Solid Edge part; units mm, degrees
sketch "Sketch1" plane through (0, 0, 0) normal (0, 0, 1) x (1, 0, 0)
  line L0 (40, -40) -> (40, 40)
  line L1 (40, 40) -> (-40, 40)
  line L2 (-40, 40) -> (-40, -40)
  line L3 (-40, -40) -> (40, -40)
extrude "Protrusion1" add sketch "Sketch1" along normal blind 700
extrude "Extrusionsausschnitt_1" [suppressed]
sketch "Sketch2" plane through (40, 0, 350) normal (1, 0, 0) x (0, 0, 1)
  circle A0 centre (250, 79.99) radius 60
  circle A1 centre (250, 79.99) radius 41.1
extrude "Protrusion2" add sketch "Sketch2" against normal up to vertex (80 mm away)
sketch "Sketch3" plane through (40, -55, 350) normal (1, 0, 0) x (0, 0, 1)
  line L0 (190, 5) -> (160, 5)
  line L1 (160, 5) -> (160, -15)
  line L2 (160, -15) -> (218.8953, -15)
  line L3 (218.8953, -15) -> (190, 24.99)
  line L4 (190, 24.99) -> (190, 5)
extrude "Protrusion3" add sketch "Sketch3" against normal up to vertex (80 mm away)
mirror "Mirror1" about plane through (0, 0, 600) normal (0, 0, 1) of "Protrusion3"
hole "Bohrung_1" [suppressed]
hole "Hole1" [suppressed]
mirror "Mirror2" [suppressed]
sketch "Sketch4" plane through (0, 0, 700) normal (0, 0, 1) x (-1, 0, 0)
  circle A0 centre (0, 0) radius 5
extrude "Extrusionsausschnitt_2" cut sketch "Sketch4" against normal blind 36.6109
sketch "Sketch5" plane through (40, -55, 350) normal (1, 0, 0) x (0, 0, -1)
  line L0 (-350, 95) -> (350, 95)
  line L1 (350, 95) -> (350, 15)
  line L2 (350, 15) -> (-350, 15)
  line L3 (-350, 15) -> (-350, 95)
extrude "Extrusionsausschnitt_3" cut sketch "Sketch5" against normal blind 305.8385
sketch "Sketch6" plane through (40, -89.995, 600) normal (1, 0, 0) x (0, 0, 1)
  line L0 (41.1, -65.4793) -> (41.1, -10.005)
  line L1 (41.1, -10.005) -> (-41.1, -10.005)
  line L2 (-41.1, -10.005) -> (-41.1, -65.4793)
  line L3 (-41.1, -65.4793) -> (41.1, -65.4793)
extrude "Extrusionsausschnitt_4" cut sketch "Sketch6" against normal blind 204.5794
hole "Bohrung_3" at (20, -60, 525) direction (0, 1, 0) diameter 7 end up to next
hole "Hole2" at (-20, -60, 525) direction (0, 1, 0) diameter 7 end up to next
mirror "Mirror3" about plane through (0, 0, 600) normal (0, 0, 1) of "Bohrung_3", "Hole2"
fillet "Verrundung_1" radius 7 8 edges at (0, -40, 641.1) (0, -40, 690) (0, -60, 690) (0, -60, 540) (0, -60, 510) (0, -40, 510) (0, -40, 558.9) (0, -60, 660)
chamfer "Fase_1" distance 0.5 angle 45 40 edges at (40, -40, 534.45) (40, -42.0503, 556.8497) (40, -63.495, 558.9) (40, -121.09, 600) (40, -63.495, 641.1) (40, -42.0503, 643.1503) (40, -40, 665.55) (40, -42.0503, 687.9497) (40, -50, 690) (40, -57.9497, 687.9497) (40, -60, 675) (40, -62.0503, 662.0503) (40, -73.495, 660) (40, -139.99, 600) (40, -73.495, 540) (40, -62.0503, 537.9497) (40, -60, 525) (40, -57.9497, 512.0503) (40, -50, 510) (40, -42.0503, 512.0503) (-40, -63.495, 558.9) (-40, -42.0503, 556.8497) (-40, -40, 534.45) (-40, -42.0503, 512.0503) (-40, -50, 510) (-40, -57.9497, 512.0503) (-40, -60, 525) (-40, -62.0503, 537.9497) (-40, -73.495, 540) (-40, -139.99, 600) (-40, -73.495, 660) (-40, -62.0503, 662.0503) (-40, -60, 675) (-40, -57.9497, 687.9497) (-40, -50, 690) (-40, -42.0503, 687.9497) (-40, -40, 665.55) (-40, -42.0503, 643.1503) (-40, -63.495, 641.1) (-40, -121.09, 600)
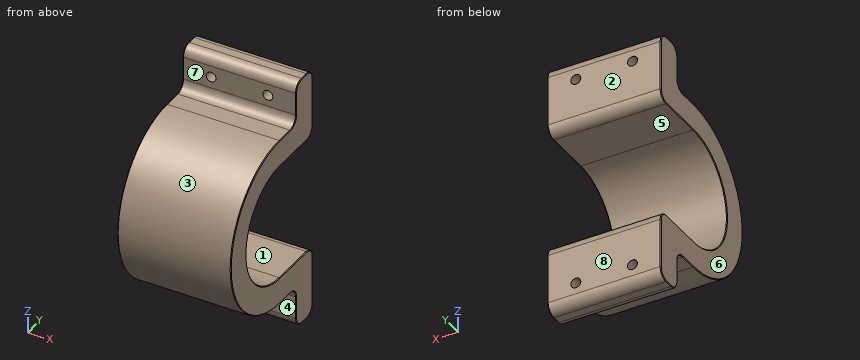
Part model, mm, in its own coordinate system. Face numbers are marked on the shaded views. A direction names the side the tool comes from. Round coordinates to 2 decimals unless told otherwise and drop trailing zeros. Loops run counter-clockwise (first coordinate to the right, second up) from the corner with the lowest first, then second, coordinate; pieces in that order, holes last. Notation, with made-up numbers: (-36.5, 0.25) -> (-0.5, 0.25) arc R14 ccw to (-0.5, 26.25) -> close; hole circle Ø5 at (-33, -24.75). An arc over 180 degrees is marked (long way). Use one line per item in the form item = value. Start each with the question number.
Item 1: Band-saw the part on B-B (z = 675). List the corners of the cut face in (x, y).
Item 2: Drill centre lines: line 1 along X through (y, z) = (-54, 525); line 2 along Z through (x, y) = (-20, -49); line 3 along Z through (x, y) = (19.5, -78). Where is each one in solid material? Low to high.
Item 3: Band-saw the part on C-C (x = -29.5). List the corners of the cut face in (y, z), plus the area to 3 significant figures.
Item 4: Band-saw the part on A-A (x = 20). List the corners of the cut face in (y, z), plus the area to 3 significant figures.
Item 5: Drop flat-ended pins along their axis: pin 1 Ø5 at (x, z) = (15, 565) entering from -Y; pin 2 Ø4 at (x, y) = (12, -73) entering from -Z; pin 3 Ø4 at (x, z) = (20, 675) entering from +Y; pin 4 Ø6 at (x, y) = (-8.5, -61) entering from +Z. Give the stop position or say it passes through.
Item 6: Two-plate mould, pull along Z, no slides. Class the marked faces 1, 2 and 3: released by +Z, released by -Z, zero draft, split by the parting line, or undercut.
Item 7: Tool access for the marked faces 4, 5, 6, 7 and 8: list every direction of +Z, -Z, +X, -X, +Y, -Y with a clear straight run to the whole face (end or side of a thin tool).
Data:
q1.outline = (-40, -59.5) -> (-39.5, -60) -> (-23.5, -60) -> (-23.5, -40) -> (-39.5, -40) -> (-40, -40.5) -> close; (-16.5, -60) -> (16.5, -60) -> (16.5, -40) -> (-16.5, -40) -> close; (23.5, -60) -> (39.5, -60) -> (40, -59.5) -> (40, -40.5) -> (39.5, -40) -> (23.5, -40) -> close
q2.line_1 = -40 to -23.5, -16.5 to 16.5, 23.5 to 40
q2.line_2 = 510 to 521.5, 528.5 to 558.9, 641.1 to 671.5, 678.5 to 690
q2.line_3 = 540 to 558.9, 641.1 to 660
q3.outline = (-79.99, 540) -> (-67, 540) arc R7 cw to (-60, 533) -> (-60, 517) arc R7 ccw to (-53, 510) -> (-47, 510) arc R7 ccw to (-40, 517) -> (-40, 551.9) arc R7 ccw to (-47, 558.9) -> (-79.99, 558.9) arc R41.1 cw to (-79.99, 641.1) -> (-47, 641.1) arc R7 ccw to (-40, 648.1) -> (-40, 683) arc R7 ccw to (-47, 690) -> (-53, 690) arc R7 ccw to (-60, 683) -> (-60, 667) arc R7 cw to (-67, 660) -> (-79.99, 660) arc R60 ccw to start
q3.area = 5,670 mm^2
q4.outline = (-79.99, 540) -> (-67, 540) arc R7 cw to (-60, 533) -> (-60, 528.5) -> (-40, 528.5) -> (-40, 551.9) arc R7 ccw to (-47, 558.9) -> (-79.99, 558.9) arc R41.1 cw to (-79.99, 641.1) -> (-47, 641.1) arc R7 ccw to (-40, 648.1) -> (-40, 671.5) -> (-60, 671.5) -> (-60, 667) arc R7 cw to (-67, 660) -> (-79.99, 660) arc R60 ccw to start; (-60, 517) arc R7 ccw to (-53, 510) -> (-47, 510) arc R7 ccw to (-40, 517) -> (-40, 521.5) -> (-60, 521.5) -> close; (-60, 678.5) -> (-40, 678.5) -> (-40, 683) arc R7 ccw to (-47, 690) -> (-53, 690) arc R7 ccw to (-60, 683) -> close
q4.area = 5,390 mm^2
q5.pin_1 = -130.43
q5.pin_2 = 540
q5.pin_3 = through
q5.pin_4 = 687.9
q6.face_1 = undercut
q6.face_2 = zero draft
q6.face_3 = split by the parting line
q7.face_4 = -Z, +X, -X, -Y
q7.face_5 = +X, -X, +Y
q7.face_6 = +Z, -Z, -X, +Y, -Y
q7.face_7 = +Z, +X, -X, -Y
q7.face_8 = +Z, -Z, +X, -X, +Y
